Can you work these out from the model? Positions are in its coordinate system, mm. A direction names the side the tool comes from. Round coordinates to 2 decimals unless told otherwise and drop trailing zeros. Loops run counter-clockwise (first coordinate to the right, second up) from the corner with the lowest first, then second, coordinate; pieces in that order, holes last. Notation, with made-up numbers: (75.25, 49.25) -> (116.25, 49.25) arc R16 ccw to (116.25, 74.25) -> close; hole circle Ø11 at (43, 19). An arc over 180 degrees is marked (long way). Answer as a JSON object with one key per item and string values.
```python
from build123d import *

# Parameters (mm, degrees)
SKETCH1_W           = 30
SKETCH1_H           = 25
BOSS_EXTRUDE1_DEPTH = 25
SKETCH2_W           = 10
SKETCH2_H           = 10
CUT_EXTRUDE3_DEPTH  = 10
SKETCH4_W           = 10
SKETCH4_H           = 5
CUT_EXTRUDE4_DEPTH  = 25
SKETCH5_W           = 10
SKETCH5_H           = 10
CUT_EXTRUDE5_DEPTH  = 10
SKETCH6_W           = 20
SKETCH6_H           = 5
CUT_EXTRUDE6_DEPTH  = 25
SKETCH7_W           = 10
SKETCH7_H           = 5
CUT_EXTRUDE7_DEPTH  = 25
SKETCH8_W           = 10
SKETCH8_H           = 5
CUT_EXTRUDE8_DEPTH  = 5
SKETCH9_W           = 10
SKETCH9_H           = 5
CUT_EXTRUDE9_DEPTH  = 5


with BuildPart() as part:
    # Sketch1 → Boss-Extrude1 (new body)
    with BuildSketch(Plane.XY):
        with Locations((15, 12.5)):
            Rectangle(SKETCH1_W, SKETCH1_H)
    extrude(amount=BOSS_EXTRUDE1_DEPTH)

    # Sketch2 → Cut-Extrude3 (cut)
    with BuildSketch(Plane.XY.offset(25)):
        with Locations((5, 5)):
            Rectangle(SKETCH2_W, SKETCH2_H)
    extrude(amount=-CUT_EXTRUDE3_DEPTH, mode=Mode.SUBTRACT)

    # Sketch4 → Cut-Extrude4 (cut)
    with BuildSketch(Plane.XY.offset(25)):
        with Locations((15, 2.5)):
            Rectangle(SKETCH4_W, SKETCH4_H)
    extrude(amount=-CUT_EXTRUDE4_DEPTH, mode=Mode.SUBTRACT)

    # Sketch5 → Cut-Extrude5 (cut)
    with BuildSketch(Plane(origin=(0, 0, 0), x_dir=(-1, 0, 0), z_dir=(0, 0, -1))):
        with Locations((-5, 5)):
            Rectangle(SKETCH5_W, SKETCH5_H)
    extrude(amount=-CUT_EXTRUDE5_DEPTH, mode=Mode.SUBTRACT)

    # Sketch6 → Cut-Extrude6 (cut)
    with BuildSketch(Plane.XY.offset(25)):
        with Locations((20, 22.5)):
            Rectangle(SKETCH6_W, SKETCH6_H)
    extrude(amount=-CUT_EXTRUDE6_DEPTH, mode=Mode.SUBTRACT)

    # Sketch7 → Cut-Extrude7 (cut)
    with BuildSketch(Plane(origin=(0, 25, 0), x_dir=(1, 0, 0), z_dir=(0, 1, 0))):
        with Locations((5, -2.5)):
            Rectangle(SKETCH7_W, SKETCH7_H)
        with Locations((5, -22.5)):
            Rectangle(SKETCH7_W, SKETCH7_H)
    extrude(amount=-CUT_EXTRUDE7_DEPTH, mode=Mode.SUBTRACT)

    # Sketch8 → Cut-Extrude8 (cut)
    with BuildSketch(Plane.XY.offset(25)):
        with Locations((15, 7.5)):
            Rectangle(SKETCH8_W, SKETCH8_H)
    extrude(amount=-CUT_EXTRUDE8_DEPTH, mode=Mode.SUBTRACT)

    # Sketch9 → Cut-Extrude9 (cut)
    with BuildSketch(Plane(origin=(0, 0, 0), x_dir=(-1, 0, 0), z_dir=(0, 0, -1))):
        with Locations((-15, 7.5)):
            Rectangle(SKETCH9_W, SKETCH9_H)
    extrude(amount=-CUT_EXTRUDE9_DEPTH, mode=Mode.SUBTRACT)


solid = part.part
```
Q1. I want a section at C-C, the plane x = 4.25. Write out the boundary of the cut face in (y, z), then the cut area to 3 significant figures.
Determined:
{"outline": "(0, 10) -> (10, 10) -> (10, 5) -> (25, 5) -> (25, 20) -> (10, 20) -> (10, 15) -> (0, 15) -> close", "area": "275 mm²"}
Q2. I want a section at B-B, the plane y = 1.75. Write out the boundary of the cut face in (x, z), then the cut area to 3 significant figures.
Determined:
{"outline": "(0, 10) -> (10, 10) -> (10, 15) -> (0, 15) -> close; (20, 0) -> (30, 0) -> (30, 25) -> (20, 25) -> close", "area": "300 mm²"}
Q3. On a 3-axis mill with a long thin cutter (end or side, diameter ignored), from which of +Z, -Z, +X, -X, +Y, -Y can I reach the whole of each face in a straight line? I mean faces 5 (the flat face through (10, 2, 13)), 6 (the flat face through (20, 20, 13)), 7 (the flat face through (5, 10, 18)). Say none if no direction works.
Determined:
{"face 5": "+Z, -Z, -Y", "face 6": "+Z, -Z, +X, +Y", "face 7": "+Z, -X, -Y"}
Q4. If I drill on L1, parallel to X at y = 2.5, z = 14.5; L2, parallel to Y at x = 27, z = 17.25; L3, parallel to Y at x = 8.25, z = 17.5, over which ranges is the centre line in solid material (lowest first)? Write a range as [from, to].
Determined:
{"L1": "[0, 10], [20, 30]", "L2": "[0, 20]", "L3": "[10, 25]"}
Q5. We'd pull the mould along X, two halves only. Please class faces 1 (the flat face through (15, 5, 13)), 2 (the flat face through (30, 10, 12)), 3 (the flat face through (5, 18, 5)), 4 (the flat face through (0, 15, 12)): pulls with the +X half, pulls with the -X half, needs draft (parallel to the pull), parting line crosses it, or undercut.
Determined:
{"face 1": "undercut", "face 2": "pulls with the +X half", "face 3": "needs draft", "face 4": "pulls with the -X half"}
Q6. I'm going to push flat-ended pins straight in: pin 1 (5.5 mm diameter, centred on x = 3.5, z = 8, fed in from -Y); pin 2 (8 mm diameter, centred on x = 5, y = 5, fed in from +Z); pin 3 (4 mm diameter, centred on x = 16, z = 2.5, fed in from -Y); pin 4 (8 mm diameter, centred on x = 5.5, y = 15.5, fed in from +Z). Where does each tip first touch, or does it pass through?
Determined:
{"pin 1": "y = 0", "pin 2": "z = 15", "pin 3": "y = 10", "pin 4": "z = 20"}
Q7. I want a section at D-D, the plane y = 11. Write out the boundary of the cut face in (x, z), then the cut area to 3 significant figures.
Determined:
{"outline": "(0, 5) -> (10, 5) -> (10, 0) -> (30, 0) -> (30, 25) -> (10, 25) -> (10, 20) -> (0, 20) -> close", "area": "650 mm²"}
Q8. I want a section at A-A, the plane z = 18.25. Write out the boundary of the cut face in (x, y).
Determined:
{"outline": "(0, 10) -> (10, 10) -> (10, 5) -> (20, 5) -> (20, 0) -> (30, 0) -> (30, 20) -> (10, 20) -> (10, 25) -> (0, 25) -> close"}
